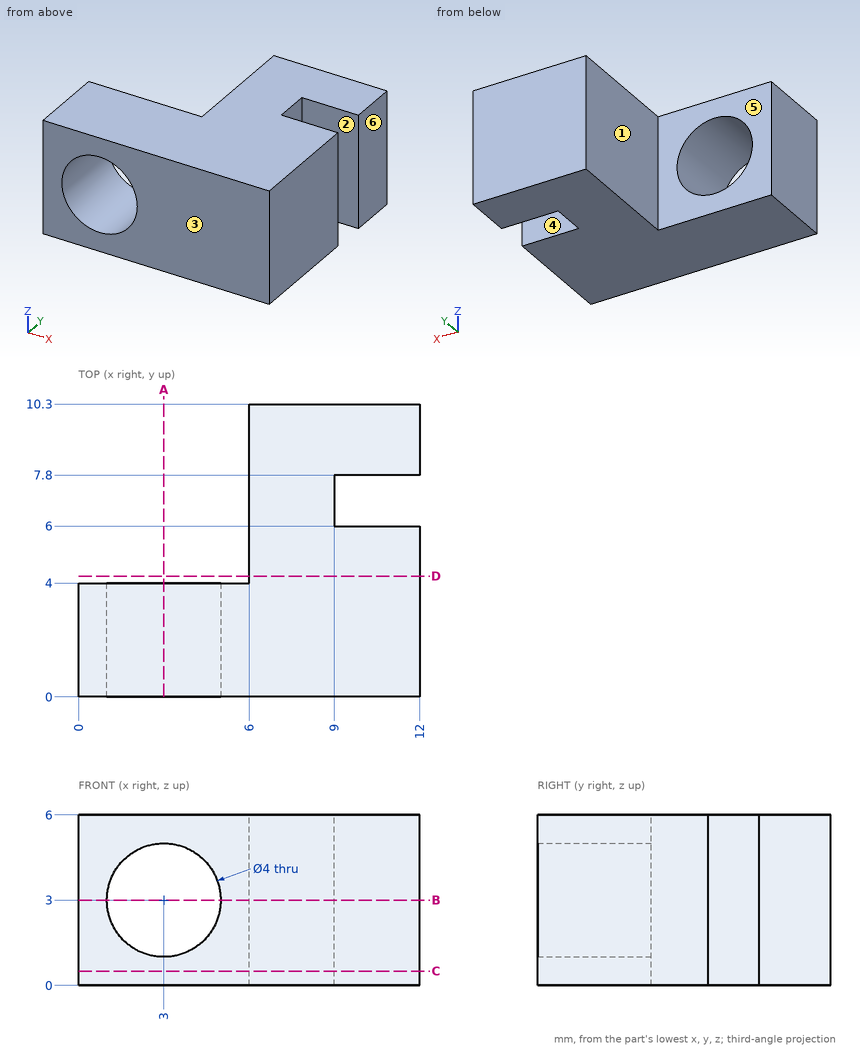
Check sheet for the drawn part. Datum: minimum x, y, z corner. Units: mm. A direction names the side the tool comes from. Round coordinates to 2 decimals unless told otherwise and drop trailing zeros. Order: outer loops, then holes, each group sorted by start corner. A loop starts at its lowest first (then second) coordinate and runs counter-clockwise, first axis right, second up. Notation, with made-up numbers: (39.25, 18) -> (60.25, 18) arc R26 ccw to (60.25, 34) -> close; hole circle Ø1 at (45.25, 73.5). An arc over 180 degrees is marked (long way). Put each result on its own line as item: value. Start each with the question number.
(1) Draft check along Y on the marked faces 4, 5 and 6. Enter one of: +Y half, -Y half, draft (parallel to the pull), parting line (faces both ways), or undercut.
(2) Depth check by flat-ended pin: pin 1 Ø3 at (x, z) = (2, 3.5) entering from +Y; pin 2 Ø0.5 at (y, z) = (7.5, 1.5) entering from +X; pin 3 Ø1 at (y, z) = (6, 4.5) entering from -X. Enter the tip coordinate at first touch or a pass-through.
(3) Tool access check on the marked faces 1, 2 and 3. Record the directions out of +Z, -Z, +X, -X, +Y, -Y that give a thin tool (end or side, any length) a straight path to the whole face; none if there is none.
(4) Section check B-B (z = 3). Enter the section's corners in (x, y), then the cut area to 3 significant figures.
(5) Section check A-A (x = 3). Enter the section's corners in (y, z).
(6) Section check C-C (z = 0.5). Enter the section's corners in (x, y).
(7) Material ranges on line 1 along X through (y, z) = (1.3, 3); line 2 along Z through (x, y) = (3, 1.2); line 3 along Y through (x, z) = (9.75, 5.5), recorded low to high.
(8) Section check D-D (y = 4.25). Enter the section's corners in (x, z).
Completed:
1. face 4: undercut
1. face 5: +Y half
1. face 6: draft
2. pin 1: stops at y = 4
2. pin 2: stops at x = 9
2. pin 3: stops at x = 6
3. face 1: +Z, -Z, -X, +Y
3. face 2: +Z, -Z, +X
3. face 3: +Z, -Z, +X, -X, -Y
4. outline: (0, 0) -> (1, 0) -> (1, 4) -> (0, 4) -> close; (5, 0) -> (12, 0) -> (12, 6) -> (9, 6) -> (9, 7.8) -> (12, 7.8) -> (12, 10.3) -> (6, 10.3) -> (6, 4) -> (5, 4) -> close
4. area: 64.4 mm2
5. outline: (0, 0) -> (4, 0) -> (4, 1) -> (0, 1) -> close; (0, 5) -> (4, 5) -> (4, 6) -> (0, 6) -> close
6. outline: (0, 0) -> (12, 0) -> (12, 6) -> (9, 6) -> (9, 7.8) -> (12, 7.8) -> (12, 10.3) -> (6, 10.3) -> (6, 4) -> (0, 4) -> close
7. line 1: x = 0 to 1, 5 to 12
7. line 2: z = 0 to 1, 5 to 6
7. line 3: y = 0 to 6, 7.8 to 10.3
8. outline: (6, 0) -> (12, 0) -> (12, 6) -> (6, 6) -> close
